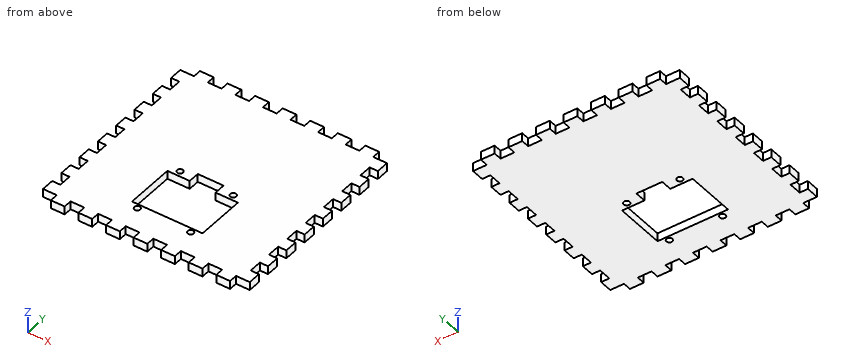
```python
from build123d import *

# Parameters (mm, degrees)
SKETCH1_W               = 80
SKETCH1_H               = 80
BOSS_EXTRUDE1_DEPTH     = 3.175
CUT_EXTRUDE2_DEPTH      = 57.657573413
CUT_EXTRUDE2_DEPTH_BACK = 57.657573413
SKETCH3_W               = 5.333333333
SKETCH3_H               = 3.175
SKETCH3_W_2             = 3.175
SKETCH3_H_2             = 4.91
SKETCH3_W_3             = 5.333333334
SKETCH4_R               = 1.15
CUT_EXTRUDE3_DEPTH      = 57.657573413


with BuildPart() as part:
    # Sketch1 → Boss-Extrude1 (new body)
    with BuildSketch(Plane.XY):
        Rectangle(SKETCH1_W, SKETCH1_H)
    extrude(amount=BOSS_EXTRUDE1_DEPTH)

    # Sketch3 → Cut-Extrude2 (cut, two sides: drawn at the far end of the back side and taken through both)
    with BuildSketch(Plane.XY.offset(3.175).offset(-CUT_EXTRUDE2_DEPTH_BACK)):
        with Locations((-37.333333334, -38.4125)):
            Rectangle(SKETCH3_W, SKETCH3_H)
        with Locations((-26.666666666, -38.4125)):
            Rectangle(SKETCH3_W, SKETCH3_H)
        with Locations((-38.4125, -29.46)):
            Rectangle(SKETCH3_W_2, SKETCH3_H_2)
        with Locations((-16, -38.4125)):
            Rectangle(SKETCH3_W_3, SKETCH3_H)
        with Locations((-38.4125, -19.64)):
            Rectangle(SKETCH3_W_2, SKETCH3_H_2)
        with Locations((-5.333333334, -38.4125)):
            Rectangle(SKETCH3_W, SKETCH3_H)
        with Locations((-38.4125, -9.82)):
            Rectangle(SKETCH3_W_2, SKETCH3_H_2)
        with Locations((5.333333334, -38.4125)):
            Rectangle(SKETCH3_W, SKETCH3_H)
        with Locations((-38.4125, 0)):
            Rectangle(SKETCH3_W_2, SKETCH3_H_2)
        with Locations((16, -38.4125)):
            Rectangle(SKETCH3_W_3, SKETCH3_H)
        with Locations((-38.4125, 9.82)):
            Rectangle(SKETCH3_W_2, SKETCH3_H_2)
        with Locations((26.666666666, -38.4125)):
            Rectangle(SKETCH3_W, SKETCH3_H)
        with Locations((-38.4125, 19.64)):
            Rectangle(SKETCH3_W_2, SKETCH3_H_2)
        with Locations((37.333333334, -38.4125)):
            Rectangle(SKETCH3_W, SKETCH3_H)
        with Locations((-38.4125, 29.46)):
            Rectangle(SKETCH3_W_2, SKETCH3_H_2)
        with Locations((-37.333333334, 38.4125)):
            Rectangle(SKETCH3_W, SKETCH3_H)
        with Locations((38.4125, -29.46)):
            Rectangle(SKETCH3_W_2, SKETCH3_H_2)
        with Locations((38.4125, -19.64)):
            Rectangle(SKETCH3_W_2, SKETCH3_H_2)
        with Locations((-26.666666666, 38.4125)):
            Rectangle(SKETCH3_W, SKETCH3_H)
        with Locations((38.4125, -9.82)):
            Rectangle(SKETCH3_W_2, SKETCH3_H_2)
        with Locations((-16, 38.4125)):
            Rectangle(SKETCH3_W_3, SKETCH3_H)
        with Locations((38.4125, 0)):
            Rectangle(SKETCH3_W_2, SKETCH3_H_2)
        with Locations((-5.333333334, 38.4125)):
            Rectangle(SKETCH3_W, SKETCH3_H)
        with Locations((38.4125, 9.82)):
            Rectangle(SKETCH3_W_2, SKETCH3_H_2)
        with Locations((5.333333334, 38.4125)):
            Rectangle(SKETCH3_W, SKETCH3_H)
        with Locations((38.4125, 19.64)):
            Rectangle(SKETCH3_W_2, SKETCH3_H_2)
        with Locations((16, 38.4125)):
            Rectangle(SKETCH3_W_3, SKETCH3_H)
        with Locations((38.4125, 29.46)):
            Rectangle(SKETCH3_W_2, SKETCH3_H_2)
        with Locations((26.666666666, 38.4125)):
            Rectangle(SKETCH3_W, SKETCH3_H)
        with Locations((37.333333334, 38.4125)):
            Rectangle(SKETCH3_W, SKETCH3_H)
    extrude(amount=CUT_EXTRUDE2_DEPTH + CUT_EXTRUDE2_DEPTH_BACK, mode=Mode.SUBTRACT)

    # Sketch4 → Cut-Extrude3 (cut, through all)
    with BuildSketch(Plane.XY.offset(3.175)):
        with Locations((-10.28, -4.475)):
            Circle(SKETCH4_R)
        with Locations((-10.3, -27.375)):
            Circle(SKETCH4_R)
        with Locations(Location((10.3, -27.375, 0), (0, 0, 180))):
            Circle(SKETCH4_R)
        with Locations(Location((10.28, -4.475, 0), (0, 0, 180))):
            Circle(SKETCH4_R)
        Polygon((5, -2.325), (5, -6.625), (13.65, -6.625), (13.65, -25.625), (-13.65, -25.625), (-13.65, -6.625), (-5, -6.625), (-5, -2.325), align=None)
    extrude(amount=-CUT_EXTRUDE3_DEPTH, mode=Mode.SUBTRACT)


solid = part.part
```
Design review of the part built by this model. Coordinates are the model's own, in mm. Give positions to 0.01 mm unless a question says otherwise; leave off trailing zeros. Write each loop counter-clockwise with the first axis right and the second up, starting at its lowest first coordinate (ties: lowest second). Pieces come first, ordered by that corner, then holes.
(1) Clearance check with flat-ended pins moving along their axes: pin 1 Ø1.6 at (x, z) = (38.5, 1.5) entering from -Y (3 decimals); pin 2 Ø1 at (x, z) = (-5.5, 1.5) entering from +Y (3 decimals); pin 3 Ø1.6 at (y, z) = (39, 1) entering from +X. State where each tip first meets the part, or that it passes through.
Checked values:
pin 1: stops at y = -36.825
pin 2: stops at y = 36.825
pin 3: stops at x = 34.67
(2) Add section C-C (y = 29.5). Give the boundary of the cut face in (x, z) (3 decimals).
Checked values:
outline: (-36.825, 0) - (36.825, 0) - (36.825, 3.175) - (-36.825, 3.175) - close
(3) Add section A-A (x = 6). Give the boundary of the cut face in (y, z) (3 decimals), and give its area (3 significant figures).
Checked values:
outline: (-36.825, 0) - (-25.625, 0) - (-25.625, 3.175) - (-36.825, 3.175) - close; (-6.625, 0) - (36.825, 0) - (36.825, 3.175) - (-6.625, 3.175) - close
area: 174 mm2
(4) Add section B-B (y = -21). Give the boundary of the cut face in (x, z) (3 decimals).
Checked values:
outline: (-36.825, 0) - (-13.65, 0) - (-13.65, 3.175) - (-36.825, 3.175) - close; (13.65, 0) - (36.825, 0) - (36.825, 3.175) - (13.65, 3.175) - close
(5) Wall thickness on line 1 along Y through (x, z) = (-10.3, 1.6) (3 decimals); line 2 along X through (y, z) = (-27.5, 1.6) (3 decimals); line 3 along X through (y, z) = (-16, 1.7): over which ranges is each line inside the solid? List them lowest first.
Checked values:
line 1: y = -40 to -28.525, -26.225 to -25.625, -6.625 to -5.625, -3.325 to 40
line 2: x = -36.825 to -11.443, -9.157 to 9.157, 11.443 to 36.825
line 3: x = -40 to -13.65, 13.65 to 40
(6) Add section D-D (z = 2.6). Give the number of separate pieces and of enclosed holes in the cut face, and give its area (3 significant figures).
Checked values:
separate pieces: 1
enclosed holes: 5
area: 5,330 mm2
